from build123d import *

# Parameters (mm, degrees)
F0_W     = 15
F0_H     = 170
F1_DEPTH = 15


with BuildPart() as f1:
    # F0 (on Front) → F1 (new body)
    with BuildSketch(Plane.XZ):
        with BuildLine():
            Line((-135, 400), (-205, 400))
            Line((-205, 400), (-205, 385))
            Line((-205, 385), (-325, 385))
            add(Edge.make_bspline(
                [(-325, 385), (-252.9975507968, 162.8222248382), (-135.9970148871, -198.2060325168), (-272.5009566468, -343.9480268474), (-325, -400)],
                knots=[0, 0, 0, 0, 0.6154027299, 1, 1, 1, 1], degree=3))
            Line((-325, -400), (-205, -400))
            ThreePointArc((-205, -400), (0, -352.0282453036), (205, -400))
            Line((205, -400), (325, -400))
            add(Edge.make_bspline(
                [(325, 385), (252.9975507968, 162.8222248382), (135.9970148871, -198.2060325168), (272.5009566468, -343.9480268474), (325, -400)],
                knots=[0, 0, 0, 0, 0.6154027299, 1, 1, 1, 1], degree=3))
            Line((325, 385), (205, 385))
            Line((205, 385), (205, 400))
            Line((205, 400), (135, 400))
            Line((135, 400), (135, 385))
            Line((135, 385), (-135, 385))
            Line((-135, 385), (-135, 400))
        make_face()
        with Locations((0, 29.998)):
            Rectangle(F0_W, F0_H, mode=Mode.SUBTRACT)
    extrude(amount=F1_DEPTH)


solid = f1.part
Read the model definition and answer for the solid it produces. Units are mm, in the model's axes. Round coordinates to 2 decimals unless told otherwise and drop trailing zeros. Loops run counter-clockwise (first coordinate to the right, second up) from the corner with the lowest first, then second, coordinate; pieces in that order, holes last. Notation, with made-up numbers: (70.5, 80.25) - (93.5, 80.25) arc R26 ccw to (93.5, 106.25) - close; hole circle Ø2 at (74.25, 22). An arc over 180 degrees is marked (long way). One line per question, with ' | ' between items. Start each with the question number.
Q1. For a pull along X with two mould halves and no side action, classify faces 1 (the flat face through (68, 0, 6)), 2 (the cylindrical face through (-2.974, -7.395, -352.038)) as +X half, -X half, draft (parallel to the pull), parting line (faces both ways), or undercut.
Q2. Section A-A on x = 28 is taken. Give the vertices of the cut face in (y, z), plus the area to 3 significant figures.
Q3. Find the intervals of material crossed by L1, parallel to Z at x = 1, y = -10.25; L2, parallel to X at y = -12, z = -4; L3, parallel to Z at x = -146.5, y = -6, in increasing order.
Q4. Section B-B on x = 147 is taken. Give the vertices of the cut face in (y, z), plus the area to 3 significant figures.
Q5. Flat-ended cylindrical pins translate along their axes: pin 1 (6 mm diameter, centred on y = -13.5, z = 68, fed in from -X); pin 2 (6 mm diameter, centred on x = -69.5, y = -2, fed in from -Z); pin 3 (7.5 mm diameter, centred on y = -10.5, z = -8.5, fed in from +X). Find the tip coordinate at first contact, or state that the pin passes through.
Established:
1) face 1: draft | face 2: undercut
2) outline: (-15, -352.88) - (0, -352.88) - (0, 385) - (-15, 385) - close | area: 11,100 mm²
3) L1: -352.03 to -55, 115 to 385 | L2: -214.85 to -7.5, 7.5 to 214.85 | L3: -375.87 to 400
4) outline: (-15, -376.04) - (0, -376.04) - (0, 400) - (-15, 400) - close | area: 11,600 mm²
5) pin 1: x = -231.18 | pin 2: z = -357.75 | pin 3: x = 214.71
